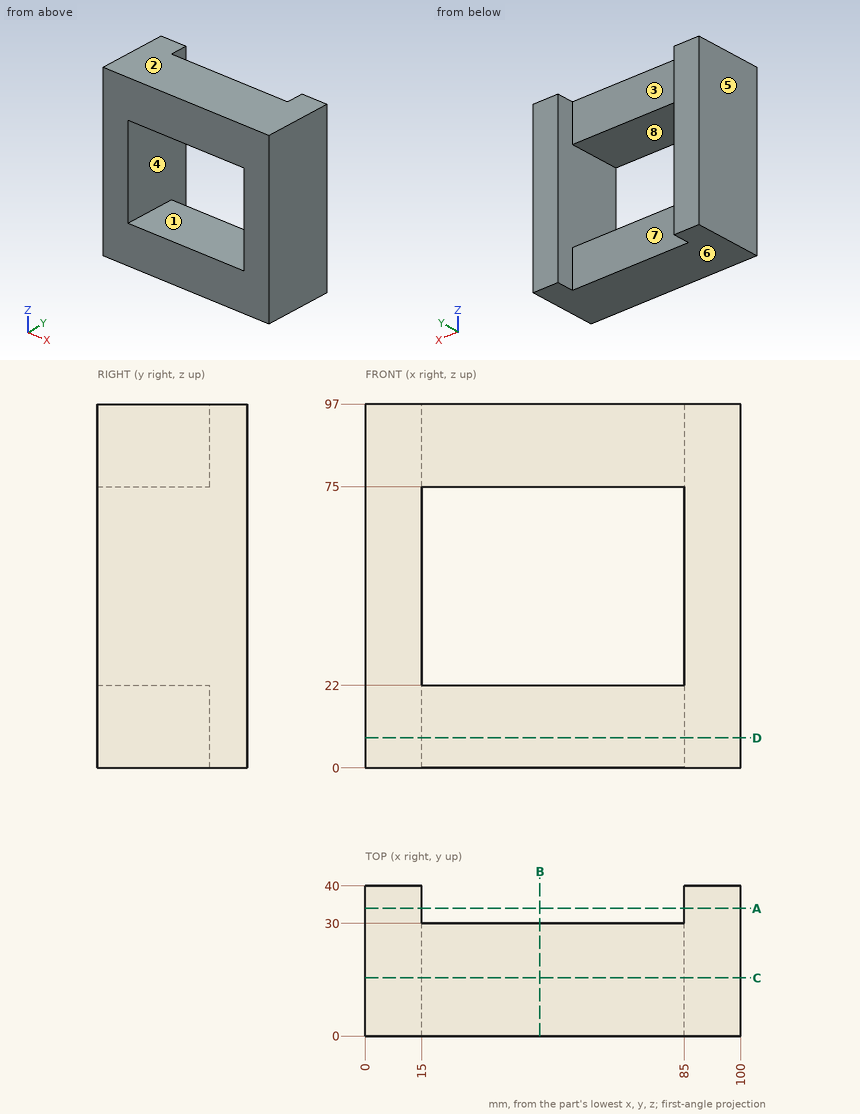
Design review of the part shown in the three views and the two pictorial views. Dimensions are in mm from the part's minimum x, y and z. A direction names the side the tool comes from. Give positions to 0.01 mm unless a question says otherwise; leave off trailing zeros. Write each loop counter-clockwise with the first axis right and the second up, starting at its lowest first coordinate (ties: lowest second). Pieces come first, ordered by that corner, then holes. Notation, with made-up numbers: (79, -8) -> (89, -8) arc R26 cw to (89, 23) -> close; hole circle Ø4 at (-36, 36). An arc over 180 degrees is marked (long way). Answer in a Markdown table with one row per item.
1) Mouldability with a two-part tool opening along Z and no side actions: class the marked faces 6, 7 and 8 as +Z half, -Z half, draft (parallel to the pull), parting line (faces both ways), or undercut.
Worked answers:
| item | result |
|---|---|
| face 6 | -Z half |
| face 7 | draft |
| face 8 | undercut |
2) Add section D-D on z = 8. State the section outline as (x, y) points, plus the area to 3 significant figures.
Worked answers:
| item | result |
|---|---|
| outline | (0, 0) -> (100, 0) -> (100, 40) -> (85, 40) -> (85, 30) -> (15, 30) -> (15, 40) -> (0, 40) -> close |
| area | 3,300 mm² |
3) Tool access review of the marked faces 1, 2, 3, 4 and 5: name each direction out of +Z, -Z, +X, -X, +Y, -Y from which nothing blocks a thin tool from reaching the whole face with its end or side.
Worked answers:
| item | result |
|---|---|
| face 1 | +Y, -Y |
| face 2 | +Z, +X, -X, +Y, -Y |
| face 3 | +Z, -Z, +Y |
| face 4 | +Y |
| face 5 | +Z, -Z, -X, +Y, -Y |
4) Clearance check with a flat-ended pin moving along its axis: P1, Ø24, axis at x = 34.5, z = 16, coming from the +Y side. State where the tip first meets the part, or that it passes through.
Worked answers:
| item | result |
|---|---|
| P1 | y = 30 |
5) Add section A-A on y = 34. State the section outline as (x, z) points.
Worked answers:
| item | result |
|---|---|
| outline | (0, 0) -> (15, 0) -> (15, 97) -> (0, 97) -> close; (85, 0) -> (100, 0) -> (100, 97) -> (85, 97) -> close |
6) Add section C-C on y = 15.5. State the section outline as (x, z) points.
Worked answers:
| item | result |
|---|---|
| outline | (0, 0) -> (100, 0) -> (100, 97) -> (0, 97) -> close; hole (15, 22) -> (85, 22) -> (85, 75) -> (15, 75) -> close |
7) For L1, parallel to X at y = 11.5, z = 67.5; L2, parallel to Z at x = 17.5, y = 13; L3, parallel to Y at x = 38, z = 11, list the stretches that pass through material, from the lowest coordinate up. Write a range as [from, to].
Worked answers:
| item | result |
|---|---|
| L1 | [0, 15], [85, 100] |
| L2 | [0, 22], [75, 97] |
| L3 | [0, 30] |
8) Add section B-B on x = 46.5. State the section outline as (y, z) points.
Worked answers:
| item | result |
|---|---|
| outline | (0, 0) -> (30, 0) -> (30, 22) -> (0, 22) -> close; (0, 75) -> (30, 75) -> (30, 97) -> (0, 97) -> close |
